from build123d import *

# Parameters (mm, degrees)
F0_W     = 101.6
F0_H     = 31.75
F1_DEPTH = 25.4
F2_R     = 9.525
F3_DEPTH = 29.90715
F4_R     = 1.6344312683
F4_R_2   = 1.5875
F4_W     = 20.6119902432
F4_H     = 38.1576609752
F5_DEPTH = 25.4
F4_H_2   = 31.75
F4_H_3   = 6.4076609752
F6_DEPTH = 2.286
F7_DEPTH = 76.2
F8_DEPTH = 6.4076609752


with BuildPart() as f1:
    # F0 (on Front) → F1 (new body)
    with BuildSketch(Plane.XZ):
        with Locations((17.1766635031, -25.9351255724)):
            Rectangle(F0_W, F0_H)
    extrude(amount=F1_DEPTH)

    # F2 (on face) → F3 (cut)
    with BuildSketch(Plane.XY.offset(-10.0601255724)):
        with Locations((-20.9235325456, -12.7)):
            Circle(F2_R)
        with Locations((0, -12.7)):
            Circle(F2_R)
        Polygon((15.4989976436, -5.0975899212), (15.4989976436, -20.6119939685), (65.0289976436, -20.6119939685), (65.0289976436, -5.0975899212), (40.2639976436, -5.0975899212), align=None)
    extrude(amount=-F3_DEPTH, mode=Mode.SUBTRACT)

    # F4 (on face) → F5 (cut)
    with BuildSketch(Plane.XZ.offset(25.4)):
        with Locations((-28.5433364969, -36.7301255724)):
            Circle(F4_R)
        with Locations((62.8966635031, -36.7301255724)):
            Circle(F4_R_2)
        with Locations((45.3453306109, -29.13895606)):
            Rectangle(F4_W, F4_H)
    extrude(amount=-F5_DEPTH, mode=Mode.SUBTRACT)

    # F4 (on face) → F6 (join)
    with BuildSketch(Plane.XZ.offset(25.4)):
        with Locations((-28.5433364969, -36.7301255724)):
            Circle(F4_R)
        with Locations((62.8966635031, -36.7301255724)):
            Circle(F4_R_2)
        with Locations((45.3453306109, -25.9351255724)):
            Rectangle(F4_W, F4_H_2)
        with Locations((45.3453306109, -45.01395606)):
            Rectangle(F4_W, F4_H_3)
    extrude(amount=-F6_DEPTH)

    # F2 (on face) → F7 (cut)
    with BuildSketch(Plane.XY.offset(-10.0601255724)):
        Polygon((15.4989976436, -5.0975899212), (15.4989976436, -20.6119939685), (65.0289976436, -20.6119939685), (65.0289976436, -5.0975899212), (40.2639976436, -5.0975899212), align=None)
    extrude(amount=-F7_DEPTH, mode=Mode.SUBTRACT)

    # F8 (cut, through all): a face of the model
    f8_faces = [f1.faces().sort_by_distance(p)[0] for p in [
        (45.3453306109, -24.257, -48.2177865475),
    ]]
    extrude(f8_faces, amount=-F8_DEPTH, mode=Mode.SUBTRACT)


solid = f1.part
Part model, mm, in its own coordinate system. A direction names the side the tool comes from. Coordinates: 2 decimals unless noted, no trailing zeros. Loops run counter-clockwise (first coordinate to the right, second up) from the corner with the lowest first, then second, coordinate; pieces in that order, holes last. Notation, with made-up numbers: (33, 83.25) -> (50, 83.25) arc R28 cw to (50, 104.25) -> close; hole circle Ø8 at (44.5, 54). An arc over 180 degrees is marked (long way). Use a Markdown table: item, result. Add a question column.
Item 1: Flat gauge pin, fed straight in: P1, Ø2.5, axis at x = -28.54, z = -36.73, coming from the +Y side. Where does the tip first touch, or does it go through?
Item 2: Probe probe 1 along Y at (x, z) = (30.5, -15); probe 2 along X at (y, z) = (-12.5, -40); probe 3 along X at (y, z) = (-11.75, -21). List the from-to ranges inside material, lowest first.
Item 3: Band-saw the part on B-B on x = 16.5. Write the cut outline in (y, z), plus the area to 3 significant figures.
Item 4: Band-saw the part on C-C on z = -22.5. Write the cut outline in (x, y) (3 decimals).
Item 5: Band-saw the part on A-A on y = -12.7. Write the cut outline in (x, z) (3 decimals), plus the area to 3 significant figures.
Item 6: Band-saw the part on D-D on x = 0. Write the cut outline in (y, z) (3 decimals).
Item 7: Which spindle directions (+Z, -Z, +X, -X, +Y, -Y) get a long thin tool onto all of the face, cutting with end or side? Do faces 4 (the cylindrical face through (-30.176, -4.137, -36.658)), 5 (the cylindrical face through (-11.84, -9.84, -24.8)), 6 (the flat face through (65.029, -13, -26)). Say none if no direction does.
Item 8: Pull direction Y, two halves, no side cores. Call faces 1 (the flat face through (-21, -13, -39.967)), 2 (the flat face through (35.039, -3, -26)), 3 (the flat face through (0, 0, -26)): +Y half, -Y half, draft (parallel to the pull), parting line (faces both ways), or undercut.
Geometry says:
| question | item | result |
|---|---|---|
| 1 | P1 | y = -23.11 |
| 2 | probe 1 | -25.4 to -20.61, -5.1 to 0 |
| 2 | probe 2 | -33.62 to 15.5, 65.03 to 67.98 |
| 2 | probe 3 | -33.62 to -30.4, -11.45 to -9.48, 9.48 to 15.5, 65.03 to 67.98 |
| 3 | outline | (-25.4, -41.81) -> (-20.61, -41.81) -> (-20.61, -10.06) -> (-25.4, -10.06) -> close; (-5.1, -41.81) -> (0, -41.81) -> (0, -10.06) -> (-5.1, -10.06) -> close |
| 3 | area | 314 mm² |
| 4 | outline | (-33.623, -25.4) -> (67.977, -25.4) -> (67.977, 0) -> (55.651, 0) -> (55.651, -5.098) -> (65.029, -5.098) -> (65.029, -20.612) -> (55.651, -20.612) -> (55.651, -23.114) -> (35.039, -23.114) -> (35.039, -20.612) -> (15.499, -20.612) -> (15.499, -5.098) -> (35.039, -5.098) -> (35.039, 0) -> (-33.623, 0) -> close; hole circle Ø19.05 at (-20.924, -12.7); hole circle Ø19.05 at (0, -12.7) |
| 5 | outline | (-33.623, -41.81) -> (15.499, -41.81) -> (15.499, -10.06) -> (9.525, -10.06) -> (9.525, -39.967) -> (-9.525, -39.967) -> (-9.525, -10.06) -> (-11.399, -10.06) -> (-11.399, -39.967) -> (-30.449, -39.967) -> (-30.449, -10.06) -> (-33.623, -10.06) -> close; (65.029, -41.81) -> (67.977, -41.81) -> (67.977, -10.06) -> (65.029, -10.06) -> close |
| 5 | area | 514 mm² |
| 6 | outline | (-25.4, -41.81) -> (0, -41.81) -> (0, -10.06) -> (-3.175, -10.06) -> (-3.175, -39.967) -> (-22.225, -39.967) -> (-22.225, -10.06) -> (-25.4, -10.06) -> close |
| 7 | face 4 | +Y |
| 7 | face 5 | +Z |
| 7 | face 6 | +Z, -Z |
| 8 | face 1 | undercut |
| 8 | face 2 | draft |
| 8 | face 3 | +Y half |
